The model under review builds one solid part; all positions refer to its coordinate system, in mm. A direction names the side the tool comes from. Coordinates: 2 decimals unless noted, no trailing zeros. Order: outer loops, then holes, each group sorted by start corner. A loop starts at its lowest first (then second) coordinate and runs counter-clockwise, first axis right, second up. Notation, with made-up numbers: (6.5, 65) -> (29.5, 65) arc R17 ccw to (29.5, 80) -> close; hole circle Ø3 at (38.25, 63). An arc over 180 degrees is marked (long way). Use CSV: the item, a comma, the result in double quotes. Start each with the question number.
```python
from build123d import *

# Parameters (mm, degrees)
EXTRUDE_1_DEPTH     = 30
SKETCH_2_R          = 2.65
CUT_EXTRUDE_1_DEPTH = 54
SKETCH_4_R          = 4.5
CUT_EXTRUDE_3_DEPTH = 40
SKETCH_5_R          = 4.25
CUT_EXTRUDE_4_DEPTH = 26
SKETCH_6_R          = 7
CUT_EXTRUDE_5_DEPTH = 8


with BuildPart() as part:
    # 草图1 → 凸台-拉伸1 (new body)
    with BuildSketch(Plane(origin=(0, 0, 0), x_dir=(0, 0, -1), z_dir=(1, 0, 0))):
        Polygon((-18.5, 8), (-18.5, -13.3), (-71.5, -13.3), (-71.5, 75), (-46.5, 75), (-46.5, 8), align=None)
    extrude(amount=EXTRUDE_1_DEPTH)

    # 草图2 → 切除-拉伸1 (cut, through all)
    with BuildSketch(Plane(origin=(0, 0, 18.5), x_dir=(-1, 0, 0), z_dir=(0, 0, -1))):
        with Locations((-15, 0)):
            Circle(SKETCH_2_R)
    extrude(amount=-CUT_EXTRUDE_1_DEPTH, mode=Mode.SUBTRACT)

    # 草图4 → 切除-拉伸3 (cut, through all)
    with BuildSketch(Plane(origin=(0, 0, 32.5), x_dir=(-1, 0, 0), z_dir=(0, 0, -1))):
        with Locations((-15, 0)):
            Circle(SKETCH_4_R)
    extrude(amount=-CUT_EXTRUDE_3_DEPTH, mode=Mode.SUBTRACT)

    # 草图5 → 切除-拉伸4 (cut, through all)
    with BuildSketch(Plane(origin=(0, 0, 46.5), x_dir=(-1, 0, 0), z_dir=(0, 0, -1))):
        with Locations((-15, 59.038200963)):
            Circle(SKETCH_5_R)
    extrude(amount=-CUT_EXTRUDE_4_DEPTH, mode=Mode.SUBTRACT)

    # 草图6 → 切除-拉伸5 (cut)
    with BuildSketch(Plane(origin=(0, 0, 46.5), x_dir=(-1, 0, 0), z_dir=(0, 0, -1))):
        with Locations((-15, 59.038200963)):
            Circle(SKETCH_6_R)
    extrude(amount=-CUT_EXTRUDE_5_DEPTH, mode=Mode.SUBTRACT)


solid = part.part
```
Q1. Draft analysis for pull direction X (two halves, no side actions). For faces 5 (the flat face through (15, -5, 18.5)), 6 (the flat face through (30, 22, 56)), 7 (the cylindrical face through (16.5, 52.2, 50.4)), state which applies: +X half, -X half, draft (parallel to the pull), parting line (faces both ways), or undercut.
Q2. For faces 1 (the flat face through (15, 42, 46.5)), 2 (the flat face through (15, 54, 54.5)), 3 (the cylindrical face through (19.496, 0.198, 51.727)), 4 (the flat face through (15, -13.3, 45)), list the 3-axis set-ups (+Z, -Z, +X, -X, +Y, -Y) from which the entire face can be reached by the end or side of a thin tool; tool diameter is ignored.
Q3. Add section C-C, the plane x = 25. State the section outline as (y, z) points.
Q4. Add section B-B, the plane z = 23.5. State the section outline as (x, y) points.
Q5. Add section D-D, the plane y = 64.5. State the section outline as (x, z) points.
Q6. Add section A-A, the plane x = 15. State the section outline as (y, z) points.
Q7. Clearance check with flat-ended pins moving along their axes: pin 1 Ø1.5 at (x, y) = (13.5, 50) entering from -Z; pin 2 Ø8.5 at (x, z) = (22, 34) entering from +Y; pin 3 Ø7 at (x, y) = (16, 59.5) entering from -Z. State where each tip first meets the part, or that it passes through.
Q8. To check wall thickness, follow probe 1 along Y at (x, z) = (15, 23); probe 2 along Y at (x, z) = (15, 64); probe 3 along Y at (x, z) = (17.75, 63). State the ranges of each line that lie inside material, in increasing order.
Answer block:
1,face 5,"draft"
1,face 6,"+X half"
1,face 7,"undercut"
2,face 1,"-Z, +X, -X, +Y"
2,face 2,"-Z"
2,face 3,"+Z"
2,face 4,"+Z, -Z, +X, -X, -Y"
3,outline,"(-13.3, 18.5) -> (8, 18.5) -> (8, 46.5) -> (75, 46.5) -> (75, 71.5) -> (-13.3, 71.5) -> close"
4,outline,"(0, -13.3) -> (30, -13.3) -> (30, 8) -> (0, 8) -> close; hole circle Ø5.3 at (15, 0)"
5,outline,"(0, 46.5) -> (10.62, 46.5) -> (10.62, 54.5) -> (19.38, 54.5) -> (19.38, 46.5) -> (30, 46.5) -> (30, 71.5) -> (0, 71.5) -> close"
6,outline,"(-13.3, 18.5) -> (-2.65, 18.5) -> (-2.65, 32.5) -> (-4.5, 32.5) -> (-4.5, 71.5) -> (-13.3, 71.5) -> close; (2.65, 18.5) -> (8, 18.5) -> (8, 46.5) -> (52.04, 46.5) -> (52.04, 54.5) -> (54.79, 54.5) -> (54.79, 71.5) -> (4.5, 71.5) -> (4.5, 32.5) -> (2.65, 32.5) -> close; (63.29, 54.5) -> (66.04, 54.5) -> (66.04, 46.5) -> (75, 46.5) -> (75, 71.5) -> (63.29, 71.5) -> close"
7,pin 1,"stops at z = 46.5"
7,pin 2,"stops at y = 8"
7,pin 3,"stops at z = 54.5"
8,probe 1,"y = -13.3 to -2.65, 2.65 to 8"
8,probe 2,"y = -13.3 to -4.5, 4.5 to 54.79, 63.29 to 75"
8,probe 3,"y = -13.3 to -3.56, 3.56 to 55.8, 62.28 to 75"
